Here's how the part is built. I have some questions about the finished solid (model axes, mm). A direction names the side the tool comes from. Coordinates: 2 decimals unless noted, no trailing zeros. Write each loop counter-clockwise with the first axis right and the second up, starting at its lowest first coordinate (ties: lowest second). Pieces come first, ordered by that corner, then holes.
Item 1: I want a section at D-D (y = -2.5). Please give me the cut outline in (x, z), and give its area (3 significant figures).
Item 2: I'm going to push flat-ended pins straight in: P1, Ø3, axis at y = -3.5, z = 2.5, coming from the -X side; P2, Ø2, axis at x = -17, y = -2, coming from the +Z side; P3, Ø6, axis at y = 3.5, z = 6, coming from the -X side; P4, Ø2.5, axis at x = 18.5, y = 0, coming from the +Z side. Where does each tip first touch, or does it pass through?
Item 3: I want a section at C-C (z = 6.5). Please give me the cut outline in (x, y).
Item 4: I want a section at A-A (z = 1.25). Please give me the cut outline in (x, y).
Item 5: I want a section at B-B (x = -7). Please give me the cut outline in (y, z), and give its area (3 significant figures).
Item 6: Please list where these lines run through material, in increasing order: line 1 (Y direction, x = -18.5, z = 1.2); line 2 (X direction, y = -5.5, z = 5).
Item 7: If we mould it in two halves opening along Y, with no side actions, what happens to faces 1 (the face through (-6.5, 0, 12)), 2 (the face through (-10, -3.6, 12)), 3 (the face through (0.071, -6.391, 7.846))? For each: pulls with the +Y half, pulls with the -Y half, needs draft (parallel to the pull), parting line crosses it, or undercut.
Item 8: For faces 4 (the face through (14.75, 0.06, 2.99)), 5 (the face through (-14, 0, 12)), 6 (the face through (-10, 3.6, 12)), 7 (the face through (-16, -3.75, 2)), 8 (the face through (16, -3.75, 2)), which set-ups out of +Z, -Z, +X, -X, +Y, -Y let a thin tool reach every point of the face, with its end or its side?
from build123d import *

# Parameters (mm, degrees)
ESQUISSE1_W                         = 29.5
ESQUISSE1_H                         = 13
BOSS_EXTRU_1_DEPTH                  = 11.5
ESQUISSE2_W                         = 4.3
ESQUISSE2_H                         = 2.3
ENL_V_MAT_EXTRU_1_DEPTH             = 30.5
ESQUISSE3_W                         = 4.3
ESQUISSE3_H                         = 2.3
ENL_V_MAT_EXTRU_2_DEPTH             = 30.5
BOSS_EXTRU_2_DEPTH                  = 2
BOSS_EXTRU_3_DEPTH                  = 2
ESQUISSE6_W                         = 7.5
ESQUISSE6_H                         = 7.2
BOSS_EXTRU_4_DEPTH                  = 2
DIAM_TRE_DU_PER_AGE_3_2_3_2_1_D     = 3.2
DIAM_TRE_DU_PER_AGE_3_2_3_2_1_DEPTH = 13.5
BOSS_EXTRU_5_DEPTH                  = 5.05
BOSS_EXTRU_5_DEPTH_BACK             = 5.05
BOSS_EXTRU_6_DEPTH                  = 7.5
ESQUISSE11_R                        = 3.75
ENL_V_MAT_EXTRU_3_DEPTH             = 9.5


with BuildPart() as part:
    # Esquisse1 → Boss.-Extru.1 (new body)
    with BuildSketch(Plane.XY.offset(11.5)):
        Rectangle(ESQUISSE1_W, ESQUISSE1_H)
    extrude(amount=-BOSS_EXTRU_1_DEPTH)

    # Esquisse2 → Enlèv. mat.-Extru.1 (cut, through all)
    with BuildSketch(Plane(origin=(14.75, 0, 0), x_dir=(0, 0, -1), z_dir=(1, 0, 0))):
        with Locations((-9.35, -5.35)):
            Rectangle(ESQUISSE2_W, ESQUISSE2_H)
    extrude(amount=-ENL_V_MAT_EXTRU_1_DEPTH, mode=Mode.SUBTRACT)

    # Esquisse3 → Enlèv. mat.-Extru.2 (cut, through all)
    with BuildSketch(Plane(origin=(14.75, 0, 0), x_dir=(0, 0, -1), z_dir=(1, 0, 0))):
        with Locations((-9.35, 5.35)):
            Rectangle(ESQUISSE3_W, ESQUISSE3_H)
    extrude(amount=-ENL_V_MAT_EXTRU_2_DEPTH, mode=Mode.SUBTRACT)

    # Esquisse4 → Boss.-Extru.2 (add)
    with BuildSketch(Plane(origin=(0, 0, 0), x_dir=(-1, 0, 0), z_dir=(0, 0, -1))):
        with BuildLine():
            Line((-14.75, -3.75), (-14.75, 3.75))
            Line((-14.75, 3.75), (-18.5, 3.75))
            ThreePointArc((-18.5, 3.75), (-22.25, 0), (-18.5, -3.75))
            Line((-18.5, -3.75), (-14.75, -3.75))
        make_face()
    extrude(amount=-BOSS_EXTRU_2_DEPTH)

    # Esquisse5 → Boss.-Extru.3 (add)
    with BuildSketch(Plane(origin=(0, 0, 0), x_dir=(-1, 0, 0), z_dir=(0, 0, -1))):
        with BuildLine():
            Line((18.5, 3.75), (14.75, 3.75))
            Line((14.75, 3.75), (14.75, -3.75))
            Line((14.75, -3.75), (18.5, -3.75))
            ThreePointArc((18.5, -3.75), (22.25, 0), (18.5, 3.75))
        make_face()
    extrude(amount=-BOSS_EXTRU_3_DEPTH)

    # Esquisse6 → Boss.-Extru.4 (add)
    with BuildSketch(Plane.XY.offset(11.5)):
        with Locations((-10.25, 0)):
            Rectangle(ESQUISSE6_W, ESQUISSE6_H)
    extrude(amount=BOSS_EXTRU_4_DEPTH)

    # Diamètre du perçage Ø3.2 (3.2)1
    with Locations(Plane(origin=(0, 0, 0), x_dir=(-1, 0, 0), z_dir=(0, 0, -1))):
        with Locations((-18.5, 0), (18.5, 0)):
            Hole(DIAM_TRE_DU_PER_AGE_3_2_3_2_1_D / 2, depth=DIAM_TRE_DU_PER_AGE_3_2_3_2_1_DEPTH)

    # Esquisse9 → Boss.-Extru.5 (add, two sides)
    with BuildSketch(Plane(origin=(0, 0, 0), x_dir=(0, 0, -1), z_dir=(1, 0, 0))) as boss_extru_5_sk:
        Polygon((-8.51, -6.83), (-10.08, -6.83), (-10.08, -12.4), (-3.3, -12.4), (-3.3, -6.5), (-7.2, -6.5), (-7.2, -5.964667694), align=None)
    extrude(amount=BOSS_EXTRU_5_DEPTH)
    extrude(boss_extru_5_sk.sketch, amount=-BOSS_EXTRU_5_DEPTH_BACK)

    # Esquisse10 → Boss.-Extru.6 (add)
    with BuildSketch(Plane(origin=(0, 3.75, 0), x_dir=(1, 0, 0), z_dir=(0, 1, 0))):
        Polygon((14.75, -2), (14.75, -4.5), (17.25, -2), align=None)
        Polygon((-14.75, -2), (-14.75, -4.5), (-17.25, -2), align=None)
    extrude(amount=-BOSS_EXTRU_6_DEPTH)

    # Esquisse11 → Enlèv. mat.-Extru.3 (cut)
    with BuildSketch(Plane.XY.offset(11.5)):
        with Locations((18.5, 0)):
            Circle(ESQUISSE11_R)
        with Locations((-18.5, 0)):
            Circle(ESQUISSE11_R)
    extrude(amount=-ENL_V_MAT_EXTRU_3_DEPTH, mode=Mode.SUBTRACT)


solid = part.part
Answer:
1. outline: (-21.3, 0) - (21.3, 0) - (21.3, 2) - (15.7, 2) - (15.7, 3.55) - (14.75, 4.5) - (14.75, 11.5) - (-6.5, 11.5) - (-6.5, 13.5) - (-14, 13.5) - (-14, 11.5) - (-14.75, 11.5) - (-14.75, 4.5) - (-15.7, 3.55) - (-15.7, 2) - (-21.3, 2) - close
1. area: 384 mm2
2. P1: stops at x = -21.62
2. P2: stops at z = 2
2. P3: stops at x = -16.25
2. P4: passes through
3. outline: (-14.75, -6.5) - (-5.05, -6.5) - (-5.05, -12.4) - (5.05, -12.4) - (5.05, -6.5) - (14.75, -6.5) - (14.75, 6.5) - (-14.75, 6.5) - close
4. outline: (-18.5, -3.75) - (-14.75, -3.75) - (-14.75, -6.5) - (14.75, -6.5) - (14.75, -3.75) - (18.5, -3.75) arc R3.75 ccw to (18.5, 3.75) - (14.75, 3.75) - (14.75, 6.5) - (-14.75, 6.5) - (-14.75, 3.75) - (-18.5, 3.75) arc R3.75 ccw to start; hole circle Ø3.2 at (-18.5, 0); hole circle Ø3.2 at (18.5, 0)
5. outline: (-6.5, 0) - (6.5, 0) - (6.5, 7.2) - (4.2, 7.2) - (4.2, 11.5) - (3.6, 11.5) - (3.6, 13.5) - (-3.6, 13.5) - (-3.6, 11.5) - (-4.2, 11.5) - (-4.2, 7.2) - (-6.5, 7.2) - close
5. area: 144 mm2
6. line 1: y = -3.75 to -1.6, 1.6 to 3.75
6. line 2: x = -14.75 to 14.75
7. face 1: needs draft
7. face 2: pulls with the -Y half
7. face 3: undercut
8. face 4: +Z, +X
8. face 5: +Z, -X, +Y, -Y
8. face 6: +Z, +X, -X, +Y
8. face 7: +Z, -Z, -X, -Y
8. face 8: +Z, -Z, +X, -Y
